Design review of the part built by this model. Coordinates are the model's own, in mm. A direction names the side the tool comes from. Round coordinates to 2 decimals unless told otherwise and drop trailing zeros. Order: outer loops, then holes, each group sorted by start corner. A loop starts at its lowest first (then second) coordinate and runs counter-clockwise, first axis right, second up.
Solid Edge part; units mm, degrees
sketch "Sketch1" plane through (0, 0, 0) normal (0, 0, 1) x (1, 0, 0)
  line L0 (42.5, 1) -> (0, 1)
  line L1 (0, 1) -> (0, 0)
  line L2 (0, 0) -> (42.5, 0)
  line L3 (42.5, 0) -> (42.5, 1)
extrude "Protrusion1" add sketch "Sketch1" against normal blind 31
sketch "Sketch2" plane through (21.25, 1, -15.5) normal (0, 1, 0) x (1, 0, 0)
  line L0 (20, -15.5) -> (20, 15.5)
  line L1 (20, 15.5) -> (-20, 15.5)
  line L2 (-20, 15.5) -> (-20, -15.5)
  line L3 (-20, -15.5) -> (20, -15.5)
extrude "Vysunutí_2" add sketch "Sketch2" along normal blind 2
sketch "Sketch3" plane through (21.25, 3, -15.5) normal (0, 1, 0) x (1, 0, 0)
  line L0 (-22.5, -15.5) -> (22.5, -15.5)
  line L1 (22.5, -15.5) -> (22.5, 15.5)
  line L2 (22.5, 15.5) -> (-22.5, 15.5)
  line L3 (-22.5, 15.5) -> (-22.5, -15.5)
extrude "Vysunutí_3" add sketch "Sketch3" along normal blind 2
sketch "Sketch4" plane through (21.25, 3, -15.5) normal (0, 1, 0) x (1, 0, 0)
  line L0 (22.5, -20.5) -> (22.5, -15.5)
  line L1 (-22.5, -20.5) -> (22.5, -20.5)
  line L2 (-22.5, -15.5) -> (-22.5, -20.5)
extrude "Protrusion2" add sketch "Sketch4" along normal blind 2 material side at (43.8, 3, 2.5)
1) Take a section at B-B on y = 1.85. Give the boundary of the cut face in (x, z).
Results:
outline: (1.25, -31) - (41.25, -31) - (41.25, 0) - (1.25, 0) - close
2) The part is to be moulded in two halves that separate along Y. For faces 6 (the face through (43.75, 4, -13)), 7 (the face through (41.25, 2, -15)), 8 (the face through (21, 0, -15)), say which applies: released by +Y, released by -Y, zero draft, split by the parting line, or undercut.
Results:
face 6: zero draft
face 7: undercut
face 8: released by -Y
3) For faces 1 (the face through (42, 1, -15)), 2 (the face through (0, 0.5, -15.3)), 3 (the face through (23, 3, 0.2)), 4 (the face through (21, 1, 0)), 5 (the face through (1, 1, -15)), list the 3-axis set-ups (+Z, -Z, +X, -X, +Y, -Y) from which the entire face can be reached by the end or side of a thin tool; tool diameter is ignored.
Results:
face 1: +Z, -Z, +X
face 2: +Z, -Z, -X, -Y
face 3: +Z
face 4: +Z, +X, -X, -Y
face 5: +Z, -Z, -X
4) To check wall thickness, follow line 1 along X through (y, z) = (2.05, -19); line 2 along X through (y, z) = (0.3, -13.5); line 3 along Z through (x, y) = (18.5, 1.75). State the ranges of each line that lie inside material, in increasing order.
Results:
line 1: x = 1.25 to 41.25
line 2: x = 0 to 42.5
line 3: z = -31 to 0
5) Take a section at C-C on x = 30. Give the boundary of the cut face in (y, z), plus the area to 3 significant figures.
Results:
outline: (0, -31) - (5, -31) - (5, 5) - (3, 5) - (3, 0) - (0, 0) - close
area: 165 mm2
6) Clearance check with flat-ended pins moving along their axes: P1, Ø2.5, axis at x = 16, y = 1, coming from the +Z side; P2, Ø1.6, axis at y = 1.5, z = -17.5, coming from the -X side; P3, Ø0.5, axis at y = 0.5, z = -23, coming from the +X side. State where each tip first meets the part, or that it passes through.
Results:
P1: stops at z = 0
P2: stops at x = 0
P3: stops at x = 42.5
7) Take a section at A-A on z = -26. Give the boundary of the cut face in (x, y), plus the area to 4 significant figures.
Results:
outline: (-1.25, 3) - (1.25, 3) - (1.25, 1) - (0, 1) - (0, 0) - (42.5, 0) - (42.5, 1) - (41.25, 1) - (41.25, 3) - (43.75, 3) - (43.75, 5) - (-1.25, 5) - close
area: 212.5 mm2
